Design review of the part shown in the three views and the two pictorial views. Dimensions are in mm from the part's minimum x, y and z. A direction names the side the tool comes from. Round coordinates to 2 decimals unless told otherwise and drop trailing zeros. Order: outer loops, then holes, each group sorted by start corner. A loop starts at its lowest first (then second) coordinate and runs counter-clockwise, first axis right, second up.
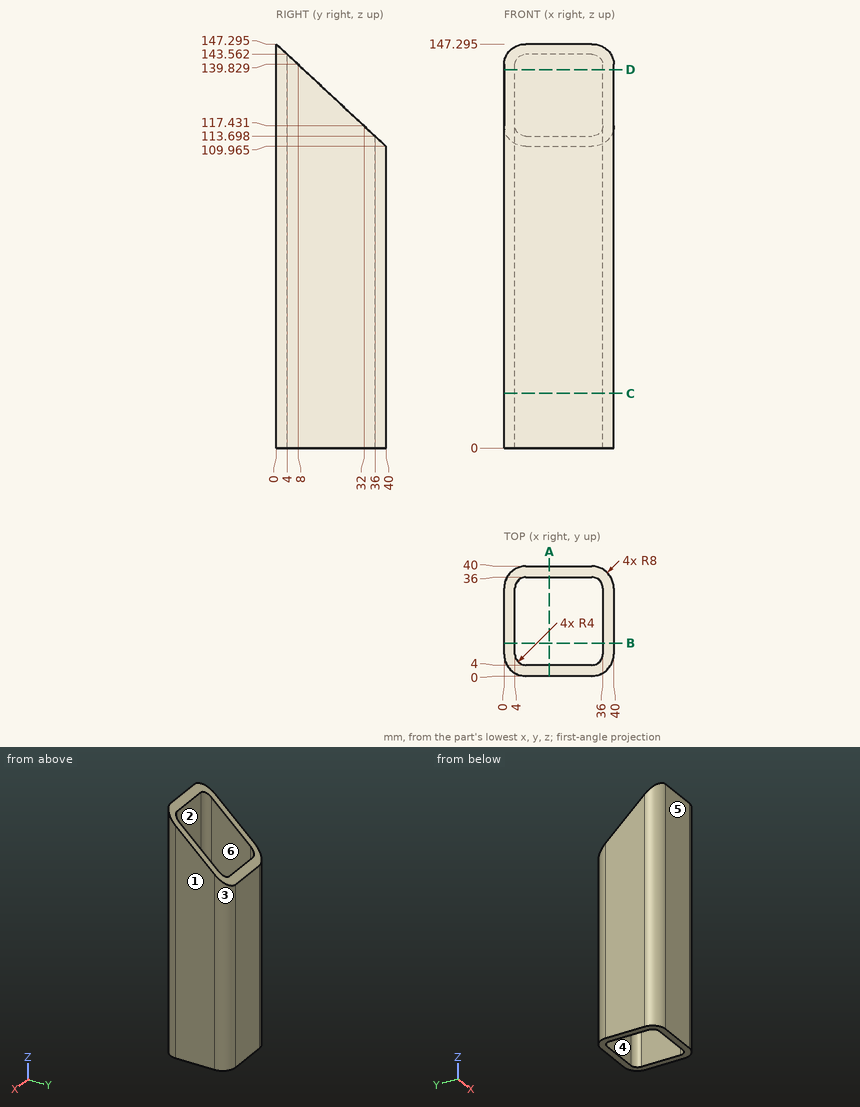
(1) Consider section B-B (y = 12). Write out the cut boundary in (x, z).
Data:
outline: (0, 0) - (4, 0) - (4, 136.1) - (0, 136.1) - close; (36, 0) - (40, 0) - (40, 136.1) - (36, 136.1) - close
(2) Draft analysis for pull direction Y (two halves, no side actions). For the marked faces 1, 2, 3 and 4, state which applies: pulls with the +Y half, pulls with the -Y half, needs draft (parallel to the pull), parting line crosses it, or undercut.
Data:
face 1: needs draft
face 2: undercut
face 3: pulls with the +Y half
face 4: undercut
(3) Consider section D-D (z = 138). Write out the cut boundary in (x, y).
Data:
outline: (0, 8) arc R8 ccw to (8, 0) - (32, 0) arc R8 ccw to (40, 8) - (40, 9.96) - (36, 9.96) - (36, 8) arc R4 cw to (32, 4) - (8, 4) arc R4 cw to (4, 8) - (4, 9.96) - (0, 9.96) - close
(4) Insertion check: pin 1 (4 mm diameter, centred on x = 8.5, z = 115, fed in from +Y); pin 2 (5 mm diameter, centred on x = 4.5, z = 30, fed in from -Y). Each pin has a flat end and moves straight along its axis. Give the tip position at first contact, or say it passes through.
Data:
pin 1: stops at y = 36.75
pin 2: stops at y = 0.06
(5) For the marked faces 5 and 6, list the 3-axis set-ups (+Z, -Z, +X, -X, +Y, -Y) from which the entire face can be reached by the end or side of a thin tool; tool diameter is ignored.
Data:
face 5: +Z, -Z, +X, -X, -Y
face 6: +Z, -Z
(6) Consider section C-C (z = 20). Write out the cut boundary in (x, y), and give its area (3 significant figures).
Data:
outline: (0, 8) arc R8 ccw to (8, 0) - (32, 0) arc R8 ccw to (40, 8) - (40, 32) arc R8 ccw to (32, 40) - (8, 40) arc R8 ccw to (0, 32) - close; hole (4, 8) arc R4 ccw to (8, 4) - (32, 4) arc R4 ccw to (36, 8) - (36, 32) arc R4 ccw to (32, 36) - (8, 36) arc R4 ccw to (4, 32) - close
area: 535 mm2
(7) Consider section A-A (x = 16.5). Write out the cut boundary in (y, z) (1 decimal).
Data:
outline: (0, 0) - (4, 0) - (4, 143.6) - (0, 147.3) - close; (36, 0) - (40, 0) - (40, 110) - (36, 113.7) - close
(8) To check wall thickness, follow probe 1 along Y at (x, z) = (8, 97); probe 2 along Y at (x, z) = (6.5, 58). State the ranges of each line that lie inside material, in increasing order.
Data:
probe 1: y = 0 to 4, 36 to 40
probe 2: y = 0.14 to 4.29, 35.71 to 39.86
